Autodesk Inventor part; units mm, degrees
ref_plane "YZ Plane" through (0, 0, 0) normal (1, 0, 0) x (0, 1, 0)
ref_plane "XZ Plane" through (0, 0, 0) normal (0, 1, 0) x (-1, 0, 0)
ref_plane "XY Plane" through (0, 0, 0) normal (0, 0, 1) x (1, 0, 0)
sketch "Sketch1" plane through (0, 0, 0) normal (0, 1, 0) x (-1, 0, 0)
  circle A0 centre (0, -15) radius 2.1
  circle A1 centre (12.9904, 7.5) radius 2.1
  circle A2 centre (-12.9904, 7.5) radius 2.1
  line L0 (20.4449, 23.6603) -> (30.7128, 5.8756)
  line L1 (-20.4449, 23.6603) -> (-30.7128, 5.8756)
  line L2 (-10.2679, -29.5359) -> (10.2679, -29.5359)
  circle A3 centre (15.55, -15.55) radius 1.6
  circle A4 centre (15.55, 15.55) radius 1.6
  circle A5 centre (-15.55, 15.55) radius 1.6
  circle A6 centre (-15.55, -15.55) radius 1.6
  line L3 (30.7128, 5.8756) -> (33.2128, 1.5455)
  line L4 (-20.4449, 23.6603) -> (-17.9449, 27.9904)
  line L5 (-10.2679, -29.5359) -> (-15.2679, -29.5359)
  line L6 (10.2679, -29.5359) -> (15.2679, -29.5359)
  line L7 (20.4449, 23.6603) -> (17.9449, 27.9904)
  line L8 (-30.7128, 5.8756) -> (-33.2128, 1.5455)
  line L9 (17.9449, 27.9904) -> (-17.9449, 27.9904)
  line L10 (15.2679, -29.5359) -> (33.2128, 1.5455)
  line L11 (17.9449, 27.9904) -> (-17.9449, 27.9904)
  line L12 (-33.2128, 1.5455) -> (-15.2679, -29.5359)
  circle A7 centre (0, 0) radius 11.15
  dimension "d29" = 360
  dimension "d77" = 360
  dimension "d82" = 360
  dimension "d86" = 360
  dimension "d90" = 360
sketch "Sketch4" plane through (0, 0, 0) normal (0, 1, 0) x (-1, 0, 0)
  point P0 (0, 0)
extrude "Extrusion5" add sketch "Sketch1" along normal blind 3
chamfer "Chamfer6" distance 0.5 angle 45 1 edges at (11.15, 3, 0)
chamfer "Chamfer7" distance 0.2 angle 45 3 edges at (-10.8904, 3, 7.5) (2.1, 3, -15) (15.0904, 3, 7.5)
fillet "Fillet1" radius 2 6 edges at (17.9449, 1.5, 27.9904) (33.2128, 1.5, 1.5455) (15.2679, 1.5, -29.5359) (-15.2679, 1.5, -29.5359) (-33.2128, 1.5, 1.5455) (-17.9449, 1.5, 27.9904)
chamfer "Chamfer8" distance 0.5 angle 45 12 edges at (-24.2404, 3, -13.9952) (-32.9034, 3, 1.5455) (-25.5788, 3, 14.7679) (-17.7902, 3, 27.7224) (0, 3, 27.9904) (17.7902, 3, 27.7224) (25.5788, 3, 14.7679) (32.9034, 3, 1.5455) (24.2404, 3, -13.9952) (15.1132, 3, -29.2679) (0, 3, -29.5359) (-15.1132, 3, -29.2679)
properties part number "4_DOF"
Work out the finished part from the listing and answer in its coordinate system (mm). Give positions to 0.01 mm unless a question says otherwise; leave off trailing zeros. Loops run counter-clockwise (first coordinate to the right, second up) from the corner with the lowest first, then second, coordinate; pieces in that order, holes last. Notation, with made-up numbers: (-39, -21) - (-28, -21) arc R10 ccw to (-28, -5) - close; hole circle Ø9 at (26.25, 60). An arc over 180 degrees is marked (long way). Use CSV: the item, a comma, the result in double quotes. Start each with the question number.
(1) Find section B-B, the plane y = 1.2. Count the separate pieces of the cut face and the enclosed holes in it, plus the area to 3 significant figures.
(2) Find section A-A, the plane x = 0. Determine the outline of the cut face in (y, z).
(3) Find the intervals of material crossed by L1, parallel to Z at x = 0, y = 1.4; L2, parallel to Z at x = -15.55, y = 1.2; L3, parallel to Z at x = 10, y = 2.15, in increasing order.
(4) Find section D-D, the plane x = -22. Determine the outline of the cut face in (y, z).
(5) Find section C-C, the plane z = 15.55. Determine the outline of the cut face in (x, y), plus the area to 3 significant figures.
(6) Determine the mould class of faces 1 (the face through (-32.903, 1.268, 1.531)), 2 (the face through (15.13, 1.27, -29.26)), 3 (the face through (-13.95, 1.48, -15.62)) for opening direction Z: released by +Z, released by -Z, zero draft, split by the parting line, or undercut.
Results found:
1,separate pieces,"1"
1,enclosed holes,"8"
1,area,"2,390 mm^2"
2,outline,"(0, -29.54) - (2.5, -29.54) - (3, -29.04) - (3, -17.3) - (2.8, -17.1) - (0, -17.1) - close; (0, -12.9) - (2.8, -12.9) - (3, -12.7) - (3, -11.65) - (2.5, -11.15) - (0, -11.15) - close; (0, 11.15) - (2.5, 11.15) - (3, 11.65) - (3, 27.49) - (2.5, 27.99) - (0, 27.99) - close"
3,L1,"-29.54 to -17.1, -12.9 to -11.15, 11.15 to 27.99"
3,L2,"-28.93 to -17.15, -13.95 to 13.95, 17.15 to 27.99"
3,L3,"-29.54 to -4.93, 4.93 to 27.99"
4,outline,"(0, -17.88) - (2.5, -17.88) - (3, -16.88) - (3, 19.97) - (2.5, 20.97) - (0, 20.97) - close"
5,outline,"(-25.13, 0) - (-17.15, 0) - (-17.15, 3) - (-24.55, 3) - (-25.13, 2.5) - close; (-13.95, 0) - (13.95, 0) - (13.95, 3) - (-13.95, 3) - close; (17.15, 0) - (25.13, 0) - (25.13, 2.5) - (24.55, 3) - (17.15, 3) - close"
5,area,"131 mm^2"
6,face 1,"split by the parting line"
6,face 2,"released by -Z"
6,face 3,"undercut"
